For this review, take the finished solid that the model builds, in its own axes (mm). Face numbers are marked on the shaded views. A direction names the side the tool comes from. Coordinates: 2 decimals unless noted, no trailing zeros. Loops run counter-clockwise (first coordinate to the right, second up) from the corner with the lowest first, then second, coordinate; pieces in that order, holes last.
```python
from build123d import *

# Parameters (mm, degrees)
SKETCH_1_W                   = 10
SKETCH_1_H                   = 75
EXTRUDE_2_DEPTH              = 20
SKETCH_4_W                   = 75
SKETCH_4_H                   = 20
CUT_EXTRUDE_3_DEPTH          = 2
CUT_EXTRUDE_4_DEPTH          = 2.5
CUT_EXTRUDE_5_DEPTH          = 5
SKETCH_10_W                  = 33
SKETCH_10_H                  = 5
EXTRUDE_3_DEPTH              = 70
SKETCH_11_W                  = 5
SKETCH_11_H                  = 18
EXTRUDE_4_DEPTH              = 70
SKETCH_12_W                  = 5
SKETCH_12_H                  = 18
EXTRUDE_5_DEPTH              = 70
SKETCH_13_W                  = 60
SKETCH_13_H                  = 8
CUT_EXTRUDE_6_DEPTH          = 20
SKETCH_14_W                  = 10
SKETCH_14_H                  = 21.760680977
CUT_EXTRUDE_7_DEPTH          = 20
HOLE_WIZARD_M3_1_D           = 3.4
HOLE_WIZARD_M3_1_DEPTH       = 20
HOLE_WIZARD_M3_1_CBORE_D     = 6.7
HOLE_WIZARD_M3_1_CBORE_DEPTH = 1.65
HOLE_WIZARD_M3_1_TIP         = 1.021463052


with BuildPart() as part:
    # 草图1 → 凸台-拉伸2 (new body)
    with BuildSketch(Plane(origin=(0, 0, 0), x_dir=(1, 0, 0), z_dir=(0, 1, 0))):
        with Locations((5, 37.5)):
            Rectangle(SKETCH_1_W, SKETCH_1_H)
    extrude(amount=EXTRUDE_2_DEPTH)

    # 草图4 → 切除-拉伸3 (cut)
    with BuildSketch(Plane(origin=(10, 0, 0), x_dir=(0, 0, -1), z_dir=(1, 0, 0))):
        with Locations((37.5, 10)):
            Rectangle(SKETCH_4_W, SKETCH_4_H)
    extrude(amount=-CUT_EXTRUDE_3_DEPTH, mode=Mode.SUBTRACT)

    # 草图5 → 切除-拉伸4 (cut)
    with BuildSketch(Plane(origin=(8, 0, 0), x_dir=(0, 0, -1), z_dir=(1, 0, 0))):
        with BuildLine():
            Line((65.5, 15), (38.828693451, 17.381366656))
            ThreePointArc((38.828693451, 17.381366656), (43.253920441, 14.810654795), (45, 10))
            ThreePointArc((45, 10), (43.253920441, 5.189345205), (38.828693451, 2.618633344))
            Line((38.828693451, 2.618633344), (65.5, 5))
            ThreePointArc((65.5, 5), (70.5, 10), (65.5, 15))
        make_face()
        with BuildLine():
            Line((37.5, 17.5), (36.171306549, 17.381366656))
            ThreePointArc((36.171306549, 17.381366656), (30, 10), (36.171306549, 2.618633344))
            Line((36.171306549, 2.618633344), (37.5, 2.5))
            Line((37.5, 2.5), (38.828693451, 2.618633344))
            ThreePointArc((38.828693451, 2.618633344), (43.253920441, 5.189345205), (45, 10))
            ThreePointArc((45, 10), (43.253920441, 14.810654795), (38.828693451, 17.381366656))
            Line((38.828693451, 17.381366656), (37.5, 17.5))
        make_face()
        with BuildLine():
            Line((36.171306549, 17.381366656), (9.5, 15))
            ThreePointArc((9.5, 15), (4.5, 10), (9.5, 5))
            Line((9.5, 5), (36.171306549, 2.618633344))
            ThreePointArc((36.171306549, 2.618633344), (30, 10), (36.171306549, 17.381366656))
        make_face()
    extrude(amount=-CUT_EXTRUDE_4_DEPTH, mode=Mode.SUBTRACT)

    # 草图6 → 切除-拉伸5 (cut)
    with BuildSketch(Plane(origin=(8, 0, 0), x_dir=(0, 0, -1), z_dir=(1, 0, 0))):
        Polygon((37.5, 17.5), (24.551509831, 16.343884806), (24.551509831, 3.656115194), (37.5, 2.5), (50.5, 3.660714286), (50.5, 16.339285714), align=None)
    extrude(amount=-CUT_EXTRUDE_5_DEPTH, mode=Mode.SUBTRACT)

    # 草图10 → 凸台-拉伸3 (add)
    with BuildSketch(Plane.ZY):
        with Locations((-37.5, 2.5)):
            Rectangle(SKETCH_10_W, SKETCH_10_H)
    extrude(amount=EXTRUDE_3_DEPTH)

    # 草图11 → 凸台-拉伸4 (add)
    with BuildSketch(Plane.ZY):
        with Locations((-18.5, 9)):
            Rectangle(SKETCH_11_W, SKETCH_11_H)
    extrude(amount=EXTRUDE_4_DEPTH)

    # 草图12 → 凸台-拉伸5 (add)
    with BuildSketch(Plane.ZY):
        with Locations((-56.5, 9)):
            Rectangle(SKETCH_12_W, SKETCH_12_H)
    extrude(amount=EXTRUDE_5_DEPTH)

    # 草图13 → 切除-拉伸6 (cut)
    with BuildSketch(Plane(origin=(0, 5, 0), x_dir=(1, 0, 0), z_dir=(0, 1, 0))):
        with Locations((-40, 37.5)):
            Rectangle(SKETCH_13_W, SKETCH_13_H)
    extrude(amount=-CUT_EXTRUDE_6_DEPTH, mode=Mode.SUBTRACT)

    # 草图14 → 切除-拉伸7 (cut)
    with BuildSketch(Plane(origin=(0, 5, 0), x_dir=(1, 0, 0), z_dir=(0, 1, 0))):
        with Locations((-18, 38.119659512)):
            Rectangle(SKETCH_14_W, SKETCH_14_H)
    extrude(amount=-CUT_EXTRUDE_7_DEPTH, mode=Mode.SUBTRACT)

    # M3 凹圆头螺钉的柱形沉头孔1
    with Locations(Plane(origin=(0, 10, -37.5), x_dir=(0, 0, -1), z_dir=(-1, 0, 0))):
        with Locations((0, 0)):
            CounterBoreHole(HOLE_WIZARD_M3_1_D / 2, HOLE_WIZARD_M3_1_CBORE_D / 2, HOLE_WIZARD_M3_1_CBORE_DEPTH, depth=HOLE_WIZARD_M3_1_DEPTH)
            with Locations((0, 0, -(HOLE_WIZARD_M3_1_DEPTH + HOLE_WIZARD_M3_1_TIP / 2))):  # 118° drill point
                Cone(0, HOLE_WIZARD_M3_1_D / 2, HOLE_WIZARD_M3_1_TIP, mode=Mode.SUBTRACT)


solid = part.part
```
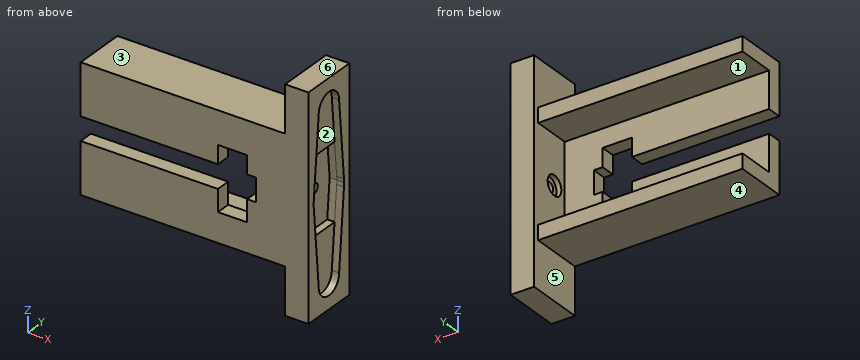
Q1. For pin 1 Ø3 at (y, z) = (12, -19.5) entering from +X; pin 2 Ø8 at (x, z) = (-47.5, -15.5) entering from +Y; pin 3 Ø3 at (x, y) = (-31.5, 12.5) entering from +Z, all flat-tipped, find the tip position at first contact; note any pin that passes through.
Q2. Machinability: for the marked faces 1, 2 and 3, which of the approach directions +Z, -Z, +X, -X, +Y, -Y give a long, thin tool a straight path to every point of the face, cutting with its end or side? Answer none if there is none.
Q3. Consider section B-B (z = -46). State the section outline as (x, y) points, then the cut area to 3 significant figures.
Q4. Consider section C-C (x = -32.5). State the section outline as (y, z) points.
Q5. Wall thickness on probe 1 along Z at (x, y) = (-18, 1.25); probe 2 along Z at (x, y) = (2.5, 10); probe 3 along Y at (x, z) = (0.9, -37.5): over which ranges is each line inside the solid? List them lowest first.
Q6. Consider section A-A (y = 10). State the section outline as (x, z) points, then the cut area to 3 significant figures.
Q7. The part is to be moulded in two halves that separate along Z. For the marked faces 4, 5 and 6, say which applies: +Z half, -Z half, draft (parallel to the pull), parting line (faces both ways), or undercut.
Q8. Consider section D-D (x = -5). State the section outline as (y, z) points.
Model answer:
1. pin 1: stops at x = 5.5
1. pin 2: stops at y = 18
1. pin 3: stops at z = -16
2. face 1: -X, +Y
2. face 2: +X
2. face 3: +Z, -X, +Y, -Y
3. outline: (-70, 0) - (-23, 0) - (-23, 5) - (-70, 5) - close; (-13, 0) - (8, 0) - (8, 3.26) - (3, 3.26) - (3, 16.74) - (8, 16.74) - (8, 20) - (0, 20) - (0, 5) - (-13, 5) - close
3. area: 393 mm2
4. outline: (0, -59) - (18, -59) - (18, -54) - (5, -54) - (5, -41.5) - (0, -41.5) - close; (0, -33.5) - (5, -33.5) - (5, -21) - (18, -21) - (18, -16) - (0, -16) - close
5. probe 1: z = -59 to -49, -27.24 to -16
5. probe 2: z = -75 to -39.2, -35.8 to 0
5. probe 3: y = 0 to 6.65, 13.35 to 20
6. outline: (-70, -59) - (0, -59) - (0, -75) - (8, -75) - (8, -70.5) - (5.5, -70.5) - (5.5, -50.5) - (3, -50.5) - (3, -39.2) - (1.65, -39.2) - (1.65, -40.85) - (0, -40.85) - (0, -54) - (-70, -54) - close; (-70, -21) - (0, -21) - (0, -34.15) - (1.65, -34.15) - (1.65, -35.8) - (3, -35.8) - (3, -24.55) - (5.5, -24.55) - (5.5, -4.5) - (8, -4.5) - (8, 0) - (0, 0) - (0, -16) - (-70, -16) - close
6. area: 1,050 mm2
7. face 4: -Z half
7. face 5: undercut
7. face 6: +Z half
8. outline: (0, -59) - (18, -59) - (18, -54) - (5, -54) - (5, -21) - (18, -21) - (18, -16) - (0, -16) - close
